from build123d import *

# Parameters (mm, degrees)
SKETCH1_R           = 5
BOSS_EXTRUDE1_DEPTH = 30
CHAMFER1_SIZE       = 0.5
CUT_EXTRUDE1_START  = -3
SKETCH2_R           = 6
SKETCH2_R_2         = 4
CUT_EXTRUDE1_DEPTH  = 1


# Read off the part's stored shape, not the designer's step: M8 Machine Threads Stud1
with BuildPart() as part:
    # Sketch1 → Boss-Extrude1 (new body)
    with BuildSketch(Plane(origin=(0, 0, 0), x_dir=(1, 0, 0), z_dir=(0, 1, 0))):
        with Locations(Location((0, 0, 0), (0, 0, 270))):
            Circle(SKETCH1_R)
    extrude(amount=BOSS_EXTRUDE1_DEPTH)

    # Chamfer1
    chamfer1_edges = [part.edges().sort_by_distance(p)[0] for p in [
        (0, 30, -5),
    ]]
    chamfer(chamfer1_edges, length=CHAMFER1_SIZE)

    # Sketch2 → Cut-Extrude1 (cut)
    with BuildSketch(Plane(origin=(0, 30, 0), x_dir=(1, 0, 0), z_dir=(0, 1, 0)).offset(CUT_EXTRUDE1_START)):
        Circle(SKETCH2_R)
        with Locations(Location((0, 0, 0), (0, 0, 270))):
            Circle(SKETCH2_R_2, mode=Mode.SUBTRACT)
    extrude(amount=-CUT_EXTRUDE1_DEPTH, mode=Mode.SUBTRACT)

    # M8 Machine Threads Stud1 outline → M8 Machine Threads Stud1 (revolve, cut)
    with BuildSketch(Plane.XY):
        Polygon((3.3095, 0), (5, 0), (5, 15), (4, 15), (4, 0.6905), align=None)
    revolve(axis=Axis((0, 0, 0), (0, 1, 0)), mode=Mode.SUBTRACT)


solid = part.part
The model under review builds one solid part; all positions refer to its coordinate system, in mm. Round coordinates to 2 decimals unless told otherwise and drop trailing zeros. Order: outer loops, then holes, each group sorted by start corner. A loop starts at its lowest first (then second) coordinate and runs counter-clockwise, first axis right, second up. Notation, with made-up numbers: (10.25, 19) -> (35.25, 19) arc R19 cw to (35.25, 50) -> close; hole circle Ø10 at (-12.5, 76). An arc over 180 degrees is marked (long way). Return JSON: item names as keys, results as strings.
1. Insertion check: P1, Ø4, axis at y = 7, z = -0.5, coming from the -X side; P2, Ø2, axis at x = 0, y = 6, coming from the +Z side; P3, Ø2, axis at x = -0.5, y = 6.5, coming from the -Z side. Each pin has a flat end and moves straight along its axis. Give the tip position at first contact, or say it passes through.
Answer block:
{"P1": "stops at x = -4", "P2": "stops at z = 4", "P3": "stops at z = -4"}
2. Take a section at D-D (y = 3.5). Write out the cut boundary in (x, z).
Answer block:
{"outline": "circle Ø8 at (0, 0)"}
3. The part is to be moulded in two halves that separate along Y. For faces 1 (the face through (-0.867, 7.745, 3.905)), 2 (the face through (-3.905, 26.507, -0.867)), 3 (the face through (0, 0, 0)), say which applies: +Y half, -Y half, draft (parallel to the pull), parting line (faces both ways), or undercut.
Answer block:
{"face 1": "draft", "face 2": "undercut", "face 3": "-Y half"}
4. Take a section at A-A (z = 0). Write out the cut boundary in (x, y), then the cut area to 3 significant figures.
Answer block:
{"outline": "(-5, 15) -> (-4, 15) -> (-4, 0.69) -> (-3.31, 0) -> (3.31, 0) -> (4, 0.69) -> (4, 15) -> (5, 15) -> (5, 26) -> (4, 26) -> (4, 27) -> (5, 27) -> (5, 29.5) -> (4.5, 30) -> (-4.5, 30) -> (-5, 29.5) -> (-5, 27) -> (-4, 27) -> (-4, 26) -> (-5, 26) -> close", "area": "267 mm²"}
5. For L1, parallel to Y at x = -1, z = 4.25; L2, parallel to Z at x = 0.25, y = 15.75; L3, parallel to Y at x = -2.5, z = 4, list the stretches that pass through material, from the lowest coordinate up. Write a range as [from, to].
Answer block:
{"L1": "y = [15, 26], [27, 30]", "L2": "z = [-4.99, 4.99]", "L3": "y = [15, 26], [27, 29.78]"}
6. Take a section at C-C (y = 21). Write out the cut boundary in (x, z), then the cut area to 3 significant figures.
Answer block:
{"outline": "circle Ø10 at (0, 0)", "area": "78.5 mm²"}
7. Take a section at B-B (x = 0). Write out the cut boundary in (y, z), then the cut area to 3 significant figures.
Answer block:
{"outline": "(0, -3.31) -> (0.69, -4) -> (15, -4) -> (15, -5) -> (26, -5) -> (26, -4) -> (27, -4) -> (27, -5) -> (29.5, -5) -> (30, -4.5) -> (30, 4.5) -> (29.5, 5) -> (27, 5) -> (27, 4) -> (26, 4) -> (26, 5) -> (15, 5) -> (15, 4) -> (0.69, 4) -> (0, 3.31) -> close", "area": "267 mm²"}
